```python
from build123d import *

# Parameters (mm, degrees)
SKETCH1_R           = 10.3
SKETCH1_R_2         = 2
BOSS_EXTRUDE1_DEPTH = 4
SKETCH2_R           = 1
CUT_EXTRUDE1_DEPTH  = 4
SKETCH3_R           = 6
SKETCH3_R_2         = 4.25
CUT_EXTRUDE2_DEPTH  = 2


with BuildPart() as part:
    # Sketch1 → Boss-Extrude1 (new body)
    with BuildSketch(Plane(origin=(0, 0, 0), x_dir=(1, 0, 0), z_dir=(0, 1, 0))):
        with Locations(Location((0, 0, 0), (0, 0, 270))):
            Circle(SKETCH1_R)
        with Locations(Location((0, 0, 0), (0, 0, 270))):
            Circle(SKETCH1_R_2, mode=Mode.SUBTRACT)
    extrude(amount=BOSS_EXTRUDE1_DEPTH)

    # Sketch2 → Cut-Extrude1 (cut)
    with BuildSketch(Plane(origin=(0, 4, 0), x_dir=(-1, 0, 0), z_dir=(0, 1, 0))):
        with Locations(Location((0, -8, 0), (0, 0, 90))):
            Circle(SKETCH2_R)
        with Locations(Location((8, 0, 0), (0, 0, 90))):
            Circle(SKETCH2_R)
        with Locations(Location((-8, 0, 0), (0, 0, 90))):
            Circle(SKETCH2_R)
        with Locations(Location((0, 8, 0), (0, 0, 90))):
            Circle(SKETCH2_R)
    extrude(amount=-CUT_EXTRUDE1_DEPTH, mode=Mode.SUBTRACT)

    # Sketch3 → Cut-Extrude2 (cut)
    with BuildSketch(Plane.XZ):
        with Locations(Location((0, 0, 0), (0, 0, 270))):
            Circle(SKETCH3_R)
        with Locations(Location((0, 0, 0), (0, 0, 270))):
            Circle(SKETCH3_R_2, mode=Mode.SUBTRACT)
    extrude(amount=-CUT_EXTRUDE2_DEPTH, mode=Mode.SUBTRACT)


solid = part.part
```
Geometry check sheet. Reference: the model listing, model coordinates, mm. A direction names the side the tool comes from. Round coordinates to 2 decimals unless told otherwise and drop trailing zeros. Write each loop counter-clockwise with the first axis right and the second up, starting at its lowest first coordinate (ties: lowest second). Pieces come first, ordered by that corner, then holes. Notation, with made-up numbers: (51.5, 65) - (102.5, 65) arc R10 ccw to (102.5, 72) - close; hole circle Ø8 at (23.5, 76.5). An arc over 180 degrees is marked (long way). Write each question's results on one line, items separated by ' | '.
(1) Sectioned sample at B-B, the plane x = 0. Enter the section's corners in (y, z), plus the area to 3 significant figures.
Computed:
outline: (0, -10.3) - (4, -10.3) - (4, -9) - (0, -9) - close; (0, -7) - (4, -7) - (4, -2) - (0, -2) - (0, -4.25) - (2, -4.25) - (2, -6) - (0, -6) - close; (0, 2) - (4, 2) - (4, 7) - (0, 7) - (0, 6) - (2, 6) - (2, 4.25) - (0, 4.25) - close; (0, 9) - (4, 9) - (4, 10.3) - (0, 10.3) - close | area: 43.4 mm^2
(2) Set-up check for faces 1 (the face through (-2, 2, 0)), 2 (the face through (4.214, 0.986, 0.553)): record each of +Z, -Z, +X, -X, +Y, -Y from which the full face is reachable in a straight line by a thin tool's end or side.
Computed:
face 1: +Y, -Y | face 2: -Y
(3) Draft check along Z on faces 3 (the face through (-10.055, 1.972, -2.233)), 4 (the face through (-1, 2, 8)), 5 (the face through (1.802, 0.986, -5.723)), 6 (the face through (-2, 4, 2)). Enter one of: pulls with the +Z half, pulls with the -Z half, needs draft (parallel to the pull), parting line crosses it, or undercut.
Computed:
face 3: parting line crosses it | face 4: undercut | face 5: undercut | face 6: needs draft
(4) Depth check by flat-ended pin: pin 1 Ø1.5 at (y, z) = (0.5, 6) entering from +X; pin 2 Ø3.5 at (x, z) = (0, 0) entering from -Y; pin 3 Ø2 at (y, z) = (3.5, -4) entering from -X. Enter the tip coordinate at first touch or a pass-through.
Computed:
pin 1: stops at x = 8.86 | pin 2: passes through | pin 3: stops at x = -9.85
(5) Thickness scan on probe 1 along X at (y, z) = (1.6, 0); probe 2 along X at (y, z) = (2.8, 0); probe 3 along Z at (x, y) = (-3.75, 0.25). Record the ranges inside material, lowest first. Write a range as from..to.
Computed:
probe 1: x = -10.3..-9, -7..-6, -4.25..-2, 2..4.25, 6..7, 9..10.3 | probe 2: x = -10.3..-9, -7..-2, 2..7, 9..10.3 | probe 3: z = -9.59..-4.68, -2..2, 4.68..9.59
(6) Sectioned sample at D-D, the plane z = 8.5. Enter the section's corners in (x, y), plus the area to 3 significant figures.
Computed:
outline: (-5.82, 0) - (-0.87, 0) - (-0.87, 4) - (-5.82, 4) - close; (0.87, 0) - (5.82, 0) - (5.82, 4) - (0.87, 4) - close | area: 39.6 mm^2
(7) Sectioned sample at C-C, the plane z = 0. Enter the section's corners in (x, y).
Computed:
outline: (-10.3, 0) - (-9, 0) - (-9, 4) - (-10.3, 4) - close; (-7, 0) - (-6, 0) - (-6, 2) - (-4.25, 2) - (-4.25, 0) - (-2, 0) - (-2, 4) - (-7, 4) - close; (2, 0) - (4.25, 0) - (4.25, 2) - (6, 2) - (6, 0) - (7, 0) - (7, 4) - (2, 4) - close; (9, 0) - (10.3, 0) - (10.3, 4) - (9, 4) - close
(8) Sectioned sample at A-A, the plane y = 1.65. Enter the section's corners in (x, z), plus the area to 3 significant figures.
Computed:
outline: circle Ø20.6 at (0, 0); circle Ø8.5 at (0, 0); hole circle Ø2 at (-8, 0); hole circle Ø12 at (0, 0); hole circle Ø4 at (0, 0); hole circle Ø2 at (0, -8); hole circle Ø2 at (0, 8); hole circle Ø2 at (8, 0) | area: 252 mm^2
